For this review, take the finished solid that the model builds, in its own axes (mm). A direction names the side the tool comes from. Round coordinates to 2 decimals unless told otherwise and drop trailing zeros. Order: outer loops, then holes, each group sorted by start corner. A loop starts at its lowest first (then second) coordinate and runs counter-clockwise, first axis right, second up. Notation, with made-up numbers: (41.5, 60.5) - (61.5, 60.5) arc R23 ccw to (61.5, 97.5) - close; hole circle Ø5 at (10.5, 52). An arc over 180 degrees is marked (long way). One line per item, written item: value.
```python
from build123d import *

# Parameters (mm, degrees)
SALIENTE_EXTRUIR1_DEPTH    = 7
CROQUIS2_7_W               = 74
CROQUIS2_7_H               = 8
SALIENTE_EXTRUIR3_DEPTH    = 27
SALIENTE_EXTRUIR5_DEPTH    = 37
CROQUIS10_R                = 1.9
CORTAR_EXTRUIR3_DEPTH      = 22
CROQUIS11_R                = 3.1
CORTAR_EXTRUIR4_DEPTH      = 6
CORTAR_EXTRUIR5_DEPTH      = 6
CORTAR_EXTRUIR6_START      = -7
CROQUIS17_W                = 8
CROQUIS17_H                = 11.32382093
CORTAR_EXTRUIR6_DEPTH      = 7
CROQUIS17_5_W              = 48
CROQUIS17_5_H              = 5
SALIENTE_EXTRUIR6_DEPTH    = 16
CORTAR_EXTRUIR8_DEPTH      = 10
CORTAR_EXTRUIR9_DEPTH      = 124.133618358
CORTAR_EXTRUIR9_DEPTH_BACK = 37
REDONDEO1_R                = 4
REDONDEO2_R                = 4
REDONDEO3_R                = 2
REDONDEO5_R                = 10


with BuildPart() as part:
    # Croquis2 → Saliente-Extruir1 (new body)
    with BuildSketch(Plane.XY):
        with BuildLine():
            Line((-47.286620614, 40.816010109), (-47.286620614, -49.183989891))
            ThreePointArc((-47.286620614, -49.183989891), (-45.236368082, -54.133737359), (-40.286620614, -56.183989891))
            Line((-40.286620614, -56.183989891), (3.713379386, -56.183989891))
            ThreePointArc((3.713379386, -56.183989891), (8.663126854, -54.133737359), (10.713379386, -49.183989891))
            Line((10.713379386, -49.183989891), (10.713379386, 40.816010109))
            Line((10.713379386, 40.816010109), (-47.286620614, 40.816010109))
        make_face()
    extrude(amount=SALIENTE_EXTRUIR1_DEPTH)

    # Croquis2_7 → Saliente-Extruir3 (add)
    with BuildSketch(Plane.XY):
        with Locations((-18.286620614, 44.816010109)):
            Rectangle(CROQUIS2_7_W, CROQUIS2_7_H)
    extrude(amount=SALIENTE_EXTRUIR3_DEPTH)

    # Croquis2_14 → Saliente-Extruir5 (add)
    with BuildSketch(Plane.XY):
        with BuildLine():
            ThreePointArc((-19.286620614, 91.616010109), (-18.286620614, 83.539831039), (-17.286620614, 91.616010109))
            Line((-17.286620614, 91.616010109), (-17.286620614, 103.616010109))
            Line((-17.286620614, 103.616010109), (-7.286620614, 103.616010109))
            Line((-7.286620614, 103.616010109), (-7.286620614, 74.616010109))
            Line((-7.286620614, 74.616010109), (18.713379386, 48.816010109))
            Line((18.713379386, 48.816010109), (-5.786620614, 48.816010109))
            Line((-5.786620614, 48.816010109), (-30.786620614, 48.816010109))
            Line((-30.786620614, 48.816010109), (-55.286620614, 48.816010109))
            Line((-55.286620614, 48.816010109), (-29.286620614, 74.616010109))
            Line((-29.286620614, 74.616010109), (-29.286620614, 103.616010109))
            Line((-29.286620614, 103.616010109), (-19.286620614, 103.616010109))
            Line((-19.286620614, 103.616010109), (-19.286620614, 91.616010109))
        make_face()
    extrude(amount=SALIENTE_EXTRUIR5_DEPTH)

    # Croquis10 → Cortar-Extruir3 (cut)
    with BuildSketch(Plane(origin=(-7.286620614, 0, 0), x_dir=(0, 0, -1), z_dir=(1, 0, 0))):
        with Locations((-9, 94.816010109)):
            Circle(CROQUIS10_R)
        with Locations((-18, 94.816010109)):
            Circle(CROQUIS10_R)
        with Locations((-27, 94.816010109)):
            Circle(CROQUIS10_R)
    extrude(amount=-CORTAR_EXTRUIR3_DEPTH, mode=Mode.SUBTRACT)

    # Croquis11 → Cortar-Extruir4 (cut)
    with BuildSketch(Plane(origin=(-7.286620614, 0, 0), x_dir=(0, 0, -1), z_dir=(1, 0, 0))):
        with Locations((-27, 94.816010109)):
            Circle(CROQUIS11_R)
        with Locations((-18, 94.816010109)):
            Circle(CROQUIS11_R)
        with Locations((-9, 94.816010109)):
            Circle(CROQUIS11_R)
    extrude(amount=-CORTAR_EXTRUIR4_DEPTH, mode=Mode.SUBTRACT)

    # Croquis12 → Cortar-Extruir5 (cut)
    with BuildSketch(Plane.ZY.offset(29.286620614)):
        Polygon((21.233161507, 94.816010109), (19.616580754, 97.616010109), (16.383419246, 97.616010109), (14.766838493, 94.816010109), (16.383419246, 92.016010109), (19.616580754, 92.016010109), align=None)
        Polygon((12.233161507, 94.816010109), (10.616580754, 97.616010109), (7.383419246, 97.616010109), (5.766838493, 94.816010109), (7.383419246, 92.016010109), (10.616580754, 92.016010109), align=None)
        Polygon((30.233161507, 94.816010109), (28.616580754, 97.616010109), (25.383419246, 97.616010109), (23.766838493, 94.816010109), (25.383419246, 92.016010109), (28.616580754, 92.016010109), align=None)
    extrude(amount=-CORTAR_EXTRUIR5_DEPTH, mode=Mode.SUBTRACT)

    # Croquis17 → Cortar-Extruir6 (cut)
    with BuildSketch(Plane.XY.offset(7).offset(CORTAR_EXTRUIR6_START)):
        with BuildLine():
            Line((10.713379386, -5.183989891), (-18.286620614, -5.183989891))
            Line((-18.286620614, -5.183989891), (-47.286620614, -5.183989891))
            Line((-47.286620614, -5.183989891), (-47.286620614, -49.183989891))
            ThreePointArc((-47.286620614, -49.183989891), (-45.236368082, -54.133737359), (-40.286620614, -56.183989891))
            Line((-40.286620614, -56.183989891), (3.713379386, -56.183989891))
            ThreePointArc((3.713379386, -56.183989891), (8.663126854, -54.133737359), (10.713379386, -49.183989891))
            Line((10.713379386, -49.183989891), (10.713379386, -5.183989891))
        make_face()
        Polygon((-18.286620614, -5.183989891), (-18.286620614, -0.860168961), (-42.286620614, -0.860168961), (-42.286620614, 6.139831039), (-47.286620614, 6.139831039), (-47.286620614, -5.183989891), align=None)
        Polygon((5.713379386, -0.860168961), (-18.286620614, -0.860168961), (-18.286620614, -5.183989891), (10.713379386, -5.183989891), (10.713379386, 6.139831039), (5.713379386, 6.139831039), align=None)
        Polygon((-18.286620614, 6.139831039), (-18.286620614, 2.639831039), (-18.286620614, -0.860168961), (5.713379386, -0.860168961), (5.713379386, 6.139831039), align=None)
        Polygon((-18.286620614, -0.860168961), (-18.286620614, 2.639831039), (-18.286620614, 6.139831039), (-42.286620614, 6.139831039), (-42.286620614, -0.860168961), align=None)
        with Locations((-51.286620614, 0.477920574)):
            Rectangle(CROQUIS17_W, CROQUIS17_H)
        with Locations((14.713379386, 0.477920574)):
            Rectangle(CROQUIS17_W, CROQUIS17_H)
    extrude(amount=CORTAR_EXTRUIR6_DEPTH, mode=Mode.SUBTRACT)

    # Croquis17_5 → Saliente-Extruir6 (add)
    with BuildSketch(Plane.XY.offset(7)):
        with Locations((-18.286620614, 8.639831039)):
            Rectangle(CROQUIS17_5_W, CROQUIS17_5_H)
    extrude(amount=SALIENTE_EXTRUIR6_DEPTH)

    # Croquis18 → Cortar-Extruir8 (cut)
    with BuildSketch(Plane.XZ.offset(-6.139831039)):
        with BuildLine():
            ThreePointArc((-27.286620614, 17), (-26.225960442, 17.439339828), (-25.786620614, 18.5))
            Line((-25.786620614, 18.5), (-27.286620614, 18.5))
            Line((-27.286620614, 18.5), (-27.286620614, 17))
        make_face()
        with BuildLine():
            Line((-27.286620614, 18.5), (-25.786620614, 18.5))
            ThreePointArc((-25.786620614, 18.5), (-28.347280786, 19.560660172), (-27.286620614, 17))
            Line((-27.286620614, 17), (-27.286620614, 18.5))
        make_face()
        with BuildLine():
            ThreePointArc((-7.786620614, 18.5), (-9.286620614, 20), (-10.786620614, 18.5))
            Line((-10.786620614, 18.5), (-9.286620614, 18.5))
            Line((-9.286620614, 18.5), (-9.286620614, 17))
            ThreePointArc((-9.286620614, 17), (-8.225960442, 17.439339828), (-7.786620614, 18.5))
        make_face()
        with BuildLine():
            Line((-9.286620614, 18.5), (-10.786620614, 18.5))
            ThreePointArc((-10.786620614, 18.5), (-10.347280786, 17.439339828), (-9.286620614, 17))
            Line((-9.286620614, 17), (-9.286620614, 18.5))
        make_face()
        with BuildLine():
            ThreePointArc((-9.286620614, 13), (-10.347280786, 12.560660172), (-10.786620614, 11.5))
            Line((-10.786620614, 11.5), (-9.286620614, 11.5))
            Line((-9.286620614, 11.5), (-9.286620614, 13))
        make_face()
        with BuildLine():
            Line((-9.286620614, 11.5), (-10.786620614, 11.5))
            ThreePointArc((-10.786620614, 11.5), (-9.286620614, 10), (-7.786620614, 11.5))
            ThreePointArc((-7.786620614, 11.5), (-8.225960442, 12.560660172), (-9.286620614, 13))
            Line((-9.286620614, 13), (-9.286620614, 11.5))
        make_face()
        with BuildLine():
            ThreePointArc((-27.286620614, 13), (-28.347280786, 10.439339828), (-25.786620614, 11.5))
            Line((-25.786620614, 11.5), (-27.286620614, 11.5))
            Line((-27.286620614, 11.5), (-27.286620614, 13))
        make_face()
        with BuildLine():
            Line((-27.286620614, 11.5), (-25.786620614, 11.5))
            ThreePointArc((-25.786620614, 11.5), (-26.225960442, 12.560660172), (-27.286620614, 13))
            Line((-27.286620614, 13), (-27.286620614, 11.5))
        make_face()
    extrude(amount=-CORTAR_EXTRUIR8_DEPTH, mode=Mode.SUBTRACT)

    # Croquis19 → Cortar-Extruir9 (cut, two sides: drawn at the far end of the back side and taken through both)
    with BuildSketch(Plane.XY.offset(37).offset(-CORTAR_EXTRUIR9_DEPTH_BACK)):
        Polygon((-52.286620614, 48.816010109), (-19.286620614, 48.816010109), (-19.286620614, 74.616010109), (-26.286620614, 74.616010109), align=None)
        Polygon((-17.286620614, 74.616010109), (-17.286620614, 48.816010109), (15.713379386, 48.816010109), (-10.286620614, 74.616010109), align=None)
    extrude(amount=CORTAR_EXTRUIR9_DEPTH + CORTAR_EXTRUIR9_DEPTH_BACK, mode=Mode.SUBTRACT)

    # Redondeo1
    redondeo1_edges = [part.edges().sort_by_distance(p)[0] for p in [
        (-10.286620614, 74.616010109, 18.5),
        (15.713379386, 48.816010109, 13.5),
        (-17.286620614, 48.816010109, 13.5),
        (-17.286620614, 74.616010109, 18.5),
        (-19.286620614, 48.816010109, 13.5),
        (-19.286620614, 74.616010109, 18.5),
        (-26.286620614, 74.616010109, 18.5),
        (-52.286620614, 48.816010109, 13.5),
    ]]
    fillet(redondeo1_edges, radius=REDONDEO1_R)

    # Redondeo2
    redondeo2_edges = [part.edges().sort_by_distance(p)[0] for p in [
        (-47.286620614, 40.816010109, 3.5),
        (10.713379386, 40.816010109, 3.5),
        (-18.286620614, 40.816010109, 7),
    ]]
    fillet(redondeo2_edges, radius=REDONDEO2_R)

    # Redondeo3
    redondeo3_edges = [part.edges().sort_by_distance(p)[0] for p in [
        (5.713379386, 8.639831039, 7),
        (-42.286620614, 8.639831039, 7),
        (-18.286620614, 11.139831039, 7),
    ]]
    fillet(redondeo3_edges, radius=REDONDEO3_R)

    # Redondeo5
    redondeo5_edges = [part.edges().sort_by_distance(p)[0] for p in [
        (-29.286620614, 74.616010109, 18.5),
        (-7.286620614, 74.616010109, 18.5),
    ]]
    fillet(redondeo5_edges, radius=REDONDEO5_R)


solid = part.part
```
Item 1: Wall thickness on line 1 (X direction, y = 67.5, z = 24); line 2 (X direction, y = 61, z = 7); line 3 (Y direction, x = 0, z = 7.5): over which ranges is each line inside the solid? List them lowest first.
Returned:
line 1: -36.46 to -33.46, -19.29 to -17.29, -3.12 to -0.12
line 2: -43.01 to -40.01, -19.29 to -17.29, 3.43 to 6.43
line 3: 6.14 to 11.82, 38.75 to 48.82, 64.41 to 67.39
Item 2: Machinability: for faces 1 (the flat face through (-26.33, 93.44, 6.56)), 2 (the flat face through (-29.287, 91, 18)), 3 (the flat face through (-13.287, 93, 28)), which of the approach directions +Z, -Z, +X, -X, +Y, -Y give a long, thin tool a straight path to every point of the face, cutting with its end or side? Answer none if there is none.
Returned:
face 1: -X
face 2: +Z, -Z, -X, +Y
face 3: +X
Item 3: Take a section at D-D (z = 3.5). Count the separate pieces of the cut face and the enclosed holes in it, plus the area to 3 significant figures.
Returned:
separate pieces: 1
enclosed holes: 2
area: 3,440 mm^2
Item 4: Take a section at B-B (y = 89). Write out the cut boundary in (x, z).
Returned:
outline: (-29.29, 0) - (-22.15, 0) - (-22.15, 37) - (-29.29, 37) - close; (-14.42, 0) - (-7.29, 0) - (-7.29, 37) - (-14.42, 37) - close
Item 5: The part is to be moulded in two halves that separate along Z. For faces 4 (the cylindrical face through (-42.89, 8.91, 7.57)), 5 (the cylindrical face through (-10.431, 74.323, 18.759)), 6 (the cylindrical face through (-10.245, 94.952, 12.097)), say which applies: +Z half, -Z half, draft (parallel to the pull), parting line (faces both ways), or undercut.
Returned:
face 4: +Z half
face 5: draft
face 6: undercut
Item 6: Take a section at A-A (x = -20.5). Write out the cut boundary in (y, z).
Returned:
outline: (6.14, 0) - (49.95, 0) - (49.95, 27) - (40.82, 27) - (40.82, 11) arc R4 cw to (36.82, 7) - (13.14, 7) arc R2 cw to (11.14, 9) - (11.14, 23) - (6.14, 23) - close; (73.49, 0) - (84.19, 0) - (84.19, 37) - (73.49, 37) - close; (91.09, 0) - (103.62, 0) - (103.62, 37) - (91.09, 37) - close; hole circle Ø3.8 at (94.82, 9); hole circle Ø3.8 at (94.82, 18); hole circle Ø3.8 at (94.82, 27)
Item 7: Take a section at C-C (y = 14.5). Write out the cut boundary in (x, z), plus the area to 3 significant figures.
Returned:
outline: (-47.29, 0) - (10.71, 0) - (10.71, 7) - (-47.29, 7) - close
area: 406 mm^2
Item 8: For P1, Ø7, axis at y = 96, z = 17.5, coming from the +X side; P2, Ø4, axis at x = -15.5, y = 8.5, coming from the +Z side; P3, Ø3, axis at x = -9.5, y = 29.5, coming from the +Z side; P4, Ø5, axis at x = 7.5, z = 14.5, coming from the -Y side, all flat-tipped, find the tip position at first contact; note any pin that passes through.
Returned:
P1: x = -7.29
P2: z = 23
P3: z = 7
P4: y = 6.14
